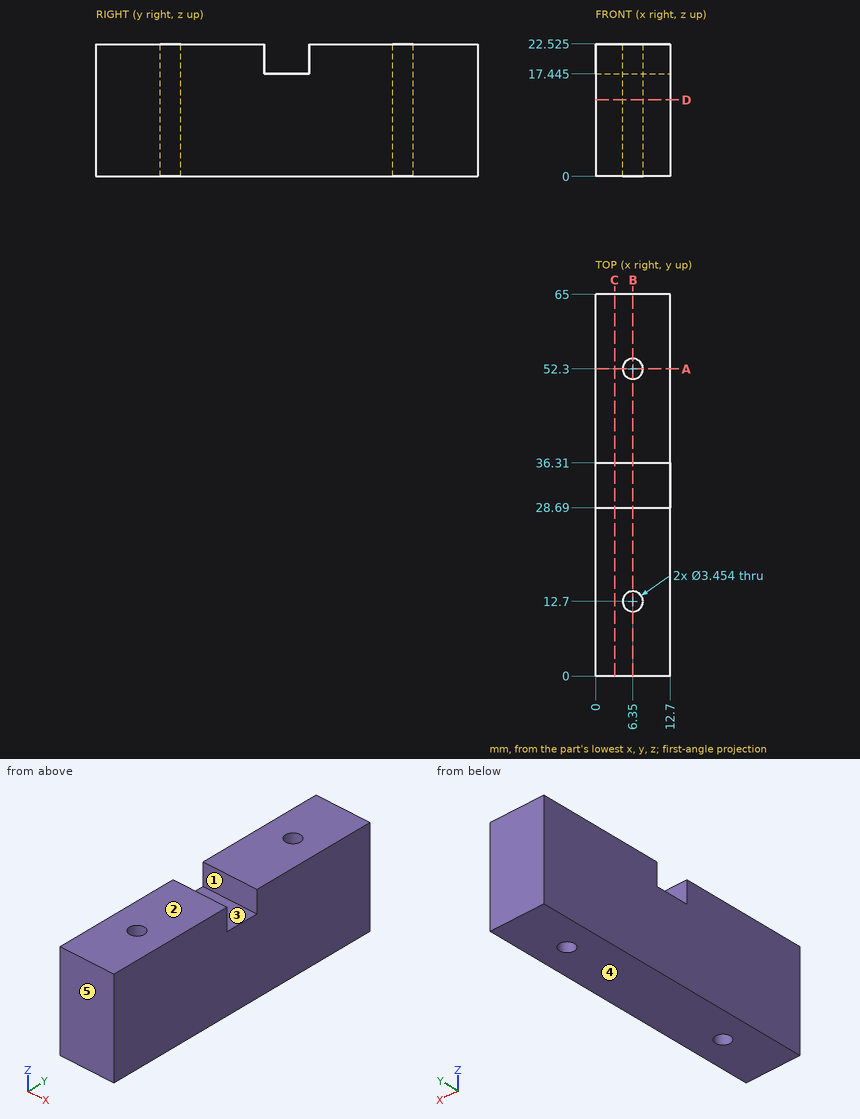
Geometry check sheet. Reference: drawing and pictorial views, mm from the part's lowest x, y, z. A direction names the side the tool comes from. Give positions to 0.01 mm unless a question says otherwise; leave off trailing zeros. Write each loop counter-clockwise with the first axis right and the second up, starting at its lowest first coordinate (ties: lowest second). Pieces come first, ordered by that corner, then holes. Notation, with made-up numbers: (24.25, 12) - (53.25, 12) arc R34 cw to (53.25, 42) - close; hole circle Ø10 at (35.25, 85.5). An arc over 180 degrees is marked (long way). Put each result on its own line as item: value.
Q1. Section check B-B on x = 6.35. Record the cut outline in (y, z) (1 decimal).
Result:
outline: (0, 0) - (11, 0) - (11, 22.5) - (0, 22.5) - close; (14.4, 0) - (50.6, 0) - (50.6, 22.5) - (36.3, 22.5) - (36.3, 17.4) - (28.7, 17.4) - (28.7, 22.5) - (14.4, 22.5) - close; (54, 0) - (65, 0) - (65, 22.5) - (54, 22.5) - close
Q2. Set-up check for the marked faces 1 and 2: record each of +Z, -Z, +X, -X, +Y, -Y from which the full face is reachable in a straight line by a thin tool's end or side.
Result:
face 1: +Z, +X, -X
face 2: +Z, +X, -X, +Y, -Y
Q3. Section check A-A on y = 52.3. Record the cut outline in (x, z) (1 decimal).
Result:
outline: (0, 0) - (4.6, 0) - (4.6, 22.5) - (0, 22.5) - close; (8.1, 0) - (12.7, 0) - (12.7, 22.5) - (8.1, 22.5) - close
Q4. Mould release check, pull along Y, two halves, no side actions. Record for the marked faces 3, 4 and 5: released by +Y, released by -Y, zero draft, split by the parting line, or undercut.
Result:
face 3: undercut
face 4: zero draft
face 5: released by -Y
Q5. Scan lines: probe 1 along Y at (x, z) = (6.35, 5.5); probe 2 along Y at (x, z) = (7.5, 12.75); probe 3 along X at (y, z) = (14, 2.5) (1 decimal). Record each from-to range of solid material in increasing order. Write a range as from..to.
Result:
probe 1: 0..10.97, 14.43..50.57, 54.03..65
probe 2: 0..11.41, 13.99..51.01, 53.59..65
probe 3: 0..5.2, 7.5..12.7
Q6. Section check C-C on x = 3.25. Record the cut outline in (y, z) (1 decimal).
Result:
outline: (0, 0) - (65, 0) - (65, 22.5) - (36.3, 22.5) - (36.3, 17.4) - (28.7, 17.4) - (28.7, 22.5) - (0, 22.5) - close
Q7. Depth check by flat-ended pin: P1, Ø3, axis at x = 6.35, y = 52.3, coming from the +Z side; P2, Ø4, axis at x = 4.5, z = 21, coming from the -Y side; P3, Ø6, axis at x = 4, y = 32, coming from the +Z side (1 decimal). Enter the tip coordinate at first touch or a pass-through.
Result:
P1: through
P2: y = 0
P3: z = 17.4
Q8. Section check D-D on z = 13. Count the separate pieces of the cut face and the enclosed holes in it, and give its area (3 significant figures).
Result:
separate pieces: 1
enclosed holes: 2
area: 807 mm2
